Here's how the part is built. I have some questions about the finished solid (model axes, mm). A direction names the side the tool comes from. Give positions to 0.01 mm unless a question says otherwise; leave off trailing zeros. Loops run counter-clockwise (first coordinate to the right, second up) from the corner with the lowest first, then second, coordinate; pieces in that order, holes last.
Q1. If we section it at B-B (x = 33.5): Please give me the cut outline in (y, z), plus the area to 3 significant figures.
Q2. If we section it at A-A (z = -14): Please give me the cut outline in (x, y).
Q3. For faces 3 (the face through (4.734, -0.74, 42.895)), 4 (the face through (42, -1, 0)), which set-ups out of +Z, -Z, +X, -X, +Y, -Y let a thin tool reach every point of the face, with its end or its side?
Q4. I need wall thicknesses on line 1 (X direction, y = -0.2, z = -33); line 2 (Z direction, x = 23.5, y = -0.75); line 3 (Z direction, x = -2, y = -0.8). Which ranges of each line are inside material? Lowest first, please.
Q5. Will these pins go through, and if not, where does the flat tip stop? P1, Ø1.2, axis at x = -37, z = 52, coming from the +Y side; P2, Ø3, axis at x = -43.5, z = -72, coming from the -Y side.
Q6. We'd pull the mould along X, two halves only. Please class faces 1 (the face through (-1, -1.5, 1)), 2 (the face through (-35.633, -0.74, -43.004)): +X half, -X half, draft (parallel to the pull), parting line (faces both ways), or undercut.
from build123d import *

# Parameters (mm, degrees)
F0_W           = 100
F0_H           = 150
F1_DEPTH       = 1.5
F3_D           = 2
F3_CSINK_D     = 4
F3_CSINK_ANGLE = 90
F4_D           = 2
F6_D           = 2


# Not quite as in the source:
# - a feature names something its author has since deleted; it is built from what else it names


with BuildPart() as f1:
    # F0 (on Front) → F1 (new body)
    with BuildSketch(Plane.XZ):
        Rectangle(F0_W, F0_H)
        with BuildLine():
            Line((-30.7377611669, -5), (-9.7377611669, -5))
            ThreePointArc((-9.7377611669, -5), (-4.7880136986, -7.0502525317), (-2.7377611669, -12))
            Line((-2.7377611669, -12), (-2.7377611669, -38))
            ThreePointArc((-2.7377611669, -38), (-4.7880136986, -42.9497474683), (-9.7377611669, -45))
            Line((-9.7377611669, -45), (-30.7377611669, -45))
            ThreePointArc((-30.7377611669, -45), (-35.6875086352, -42.9497474683), (-37.7377611669, -38))
            Line((-37.7377611669, -38), (-37.7377611669, -12))
            ThreePointArc((-37.7377611669, -12), (-35.6875086352, -7.0502525317), (-30.7377611669, -5))
        make_face(mode=Mode.SUBTRACT)
        with BuildLine():
            ThreePointArc((37.7377611669, -38), (35.6875086352, -42.9497474683), (30.7377611669, -45))
            Line((30.7377611669, -45), (9.7377611669, -45))
            ThreePointArc((9.7377611669, -45), (4.7880136986, -42.9497474683), (2.7377611669, -38))
            Line((2.7377611669, -38), (2.7377611669, -12))
            ThreePointArc((2.7377611669, -12), (4.7880136986, -7.0502525317), (9.7377611669, -5))
            Line((9.7377611669, -5), (30.7377611669, -5))
            ThreePointArc((30.7377611669, -5), (35.6875086352, -7.0502525317), (37.7377611669, -12))
            Line((37.7377611669, -12), (37.7377611669, -38))
        make_face(mode=Mode.SUBTRACT)
        with BuildLine():
            ThreePointArc((-2.7377611669, 12), (-4.7880136986, 7.0502525317), (-9.7377611669, 5))
            Line((-9.7377611669, 5), (-30.7377611669, 5))
            ThreePointArc((-30.7377611669, 5), (-35.6875086352, 7.0502525317), (-37.7377611669, 12))
            Line((-37.7377611669, 12), (-37.7377611669, 38))
            ThreePointArc((-37.7377611669, 38), (-35.6875086352, 42.9497474683), (-30.7377611669, 45))
            Line((-30.7377611669, 45), (-9.7377611669, 45))
            ThreePointArc((-9.7377611669, 45), (-4.7880136986, 42.9497474683), (-2.7377611669, 38))
            Line((-2.7377611669, 38), (-2.7377611669, 12))
        make_face(mode=Mode.SUBTRACT)
        Polygon((-24, 56.5), (-24, 68.5), (-15, 68.5), (-6, 68.5), (-6, 56.5), (-15, 56.5), align=None, mode=Mode.SUBTRACT)
        with BuildLine():
            ThreePointArc((9.7377611669, 5), (4.7880136986, 7.0502525317), (2.7377611669, 12))
            Line((2.7377611669, 12), (2.7377611669, 38))
            ThreePointArc((2.7377611669, 38), (4.7880136986, 42.9497474683), (9.7377611669, 45))
            Line((9.7377611669, 45), (30.7377611669, 45))
            ThreePointArc((30.7377611669, 45), (35.6875086352, 42.9497474683), (37.7377611669, 38))
            Line((37.7377611669, 38), (37.7377611669, 12))
            ThreePointArc((37.7377611669, 12), (35.6875086352, 7.0502525317), (30.7377611669, 5))
            Line((30.7377611669, 5), (9.7377611669, 5))
        make_face(mode=Mode.SUBTRACT)
        Polygon((6, 56.5), (6, 68.5), (15, 68.5), (24, 68.5), (24, 56.5), (15, 56.5), align=None, mode=Mode.SUBTRACT)
    extrude(amount=F1_DEPTH)

    # F3 (through all)
    with Locations(Plane.XZ.offset(1.5)):
        with Locations((-43.5, -72), (43.5, -72), (43.5, 72), (-43.5, 72), (-43.5, 0), (43.5, 0)):
            CounterSinkHole(F3_D / 2, F3_CSINK_D / 2, counter_sink_angle=F3_CSINK_ANGLE)

    # F4 (through all)
    with Locations(Plane(origin=(0, 0, 0), x_dir=(1, 0, 0), z_dir=(0, 1, 0))):
        with Locations((-28, -68), (-28, -57), (-2, -57), (-2, -68), (2, -68), (2, -57), (28, -57), (28, -68)):
            Hole(F4_D / 2)

    # F6 (through all)
    with Locations(Plane(origin=(0, 0, 0), x_dir=(1, 0, 0), z_dir=(0, 1, 0))):
        with Locations((-37, 72), (0, 72), (37, 72), (0, -52), (-37, -52), (37, -52), (-37, 0), (37, 0)):
            Hole(F6_D / 2)


solid = f1.part
Check sheet entries:
1. outline: (-1.5, -75) - (0, -75) - (0, -44.43) - (-1.5, -44.43) - close; (-1.5, -5.57) - (0, -5.57) - (0, 5.57) - (-1.5, 5.57) - close; (-1.5, 44.43) - (0, 44.43) - (0, 75) - (-1.5, 75) - close
1. area: 108 mm2
2. outline: (-50, -1.5) - (-37.74, -1.5) - (-37.74, 0) - (-50, 0) - close; (-2.74, -1.5) - (2.74, -1.5) - (2.74, 0) - (-2.74, 0) - close; (37.74, -1.5) - (50, -1.5) - (50, 0) - (37.74, 0) - close
3. face 3: +Y, -Y
3. face 4: -Y
4. line 1: x = -50 to -37.74, -2.74 to 2.74, 37.74 to 50
4. line 2: z = -75 to -45, -5 to 5, 45 to 56.5, 68.5 to 75
4. line 3: z = -75 to 56, 58 to 67, 69 to 75
5. P1: passes through
5. P2: stops at y = -1
6. face 1: draft
6. face 2: undercut
